from build123d import *


with BuildPart() as part:
    # Sketch1 → Revolve1 (revolve)
    with BuildSketch(Plane.YZ, mode=Mode.PRIVATE) as revolve1_sk:
        Polygon((0, 0), (4.8, 0), (4.8, 1.5), (3.8, 1.5), (3.8, 1.2), (2.9, 1.2), (2.9, 1.5), (-2.9, 1.5), (-2.9, 1.2), (-3.8, 1.2), (-3.8, 1.5), (-4.8, 1.5), (-4.8, 0), align=None)
    revolve(revolve1_sk.sketch.rotate(Axis((0, 4.8, 0), (0, 1, 0)), 180), axis=Axis((0, 4.8, 0), (0, 1, 0)))


solid = part.part
Model file for the job. Use its own axes, mm. Coordinates: 2 decimals unless noted, no trailing zeros. Loops run counter-clockwise (first coordinate to the right, second up) from the corner with the lowest first, then second, coordinate; pieces in that order, holes last. Notation, with made-up numbers: (17.5, 30) -> (59.5, 30) arc R17 cw to (59.5, 48) -> close; hole circle Ø5 at (29, -2.75). An arc over 180 degrees is marked (long way). Use one line per item in the form item = value. Start each with the question number.
(1) Cut at D-D on y = -2. Give the cut face in (x, z), and give its area (3 significant figures).
(2) Cut at B-B on z = 0. Give the cut face in (x, y), and give its area (3 significant figures).
(3) Probe probe 1 along Y at (x, z) = (-0.45, 1.2); probe 2 along Z at (x, y) = (-0.25, -3.25); probe 3 along X at (y, z) = (-4.25, 0.95). List the from-to ranges inside material, lowest first. Write a range as from..to.
(4) Pull direction Y, two halves, no side cores. Call faces 1 (the flat face through (0, 4.8, 0)), 2 (the cylindrical face through (-0.45, -0.04, -1.43)), 3 (the cylindrical face through (-1.01, -3.36, -0.65)), 4 (the cylindrical face through (-1.01, 3.34, -0.65)): pulls with the +Y half, pulls with the -Y half, needs draft (parallel to the pull), parting line crosses it, or undercut.
(5) Cut at A-A on x = 0. Give the cut face in (y, z), and give its area (3 significant figures).
(6) Cut at C-C on y = -3. Give the cut face in (x, z), and give its area (3 significant figures).
Values:
q1.outline = circle Ø3 at (0, 0)
q1.area = 7.07 mm2
q2.outline = (-1.5, -4.8) -> (1.5, -4.8) -> (1.5, -3.8) -> (1.2, -3.8) -> (1.2, -2.9) -> (1.5, -2.9) -> (1.5, 2.9) -> (1.2, 2.9) -> (1.2, 3.8) -> (1.5, 3.8) -> (1.5, 4.8) -> (-1.5, 4.8) -> (-1.5, 3.8) -> (-1.2, 3.8) -> (-1.2, 2.9) -> (-1.5, 2.9) -> (-1.5, -2.9) -> (-1.2, -2.9) -> (-1.2, -3.8) -> (-1.5, -3.8) -> close
q2.area = 27.7 mm2
q3.probe_1 = -4.8..-3.8, -2.9..2.9, 3.8..4.8
q3.probe_2 = -1.17..1.17
q3.probe_3 = -1.16..1.16
q4.face_1 = pulls with the +Y half
q4.face_2 = needs draft
q4.face_3 = undercut
q4.face_4 = undercut
q5.outline = (-4.8, -1.5) -> (-3.8, -1.5) -> (-3.8, -1.2) -> (-2.9, -1.2) -> (-2.9, -1.5) -> (2.9, -1.5) -> (2.9, -1.2) -> (3.8, -1.2) -> (3.8, -1.5) -> (4.8, -1.5) -> (4.8, 1.5) -> (3.8, 1.5) -> (3.8, 1.2) -> (2.9, 1.2) -> (2.9, 1.5) -> (-2.9, 1.5) -> (-2.9, 1.2) -> (-3.8, 1.2) -> (-3.8, 1.5) -> (-4.8, 1.5) -> close
q5.area = 27.7 mm2
q6.outline = circle Ø2.4 at (0, 0)
q6.area = 4.52 mm2
